```python
from build123d import *

# Parameters (mm, degrees)
F0_W     = 50.8
F0_H     = 38.1
F1_DEPTH = 12.7
F2_R     = 9.525
F3_DEPTH = 12.7


with BuildPart() as f1:
    # F0 (on Front) → F1 (new body, symmetric)
    with BuildSketch(Plane.XZ):
        with Locations((-25.4, 19.05)):
            Rectangle(F0_W, F0_H)
    extrude(amount=F1_DEPTH, both=True)

    # F2 (on face) → F3 (join)
    with BuildSketch(Plane.XY.offset(38.1)):
        with Locations((-25.677594, 0)):
            Circle(F2_R)
    extrude(amount=F3_DEPTH)


solid = f1.part
```
Geometry check sheet. Reference: the model listing, model coordinates, mm. A direction names the side the tool comes from. Round coordinates to 2 decimals unless told otherwise and drop trailing zeros. Loops run counter-clockwise (first coordinate to the right, second up) from the corner with the lowest first, then second, coordinate; pieces in that order, holes last. Notation, with made-up numbers: (79, -25) - (101, -25) arc R17 cw to (101, -20) - close; hole circle Ø3 at (48, -37.5). An arc over 180 degrees is marked (long way). Write each question's results on one line, items separated by ' | '. Start each with the question number.
Q1. Cross-section at C-C on z = 43. Enter the section's corners in (x, y) (3 decimals).
Q2. Thickness scan on line 1 (Z direction, x = -12.5, y = 0.75); line 2 (X direction, y = -8.25, z = 45.5); line 3 (X direction, y = 7, z = 41.5). Record the ranges inside material, lowest first. Write a range as [from, to].
Q3. Access from +Z, -Z, +X, -X, +Y, -Y to the whole of each face (thin tool, end or side, straight path). Record for faces 1 (the cylindrical face through (-16.592, 2.861, 44.361)), 2 (the flat face through (-26, 0, 0)).
Q4. Gauge pin test, flat ends, axial feed: P1, Ø2, axis at y = -3.5, z = 25, coming from the +X side; P2, Ø4, axis at x = -9.5, y = 6.5, coming from the +Z side. Record the tip position at first contact, or that the pin passes through.
Q5. Cross-section at D-D on x = -44. Enter the section's corners in (y, z).
Q6. Cross-section at B-B on x = -19. Enter the section's corners in (y, z), and give its area (3 significant figures).
Q7. Cross-section at A-A on y = 0. Enter the section's corners in (x, z), and give its area (3 significant figures).
Answers below:
1) outline: circle Ø19.05 at (-25.678, 0)
2) line 1: z = [0, 38.1] | line 2: x = [-30.44, -20.92] | line 3: x = [-32.14, -19.22]
3) face 1: +Z | face 2: -Z, +X, -X, +Y, -Y
4) P1: stops at x = 0 | P2: stops at z = 38.1
5) outline: (-12.7, 0) - (12.7, 0) - (12.7, 38.1) - (-12.7, 38.1) - close
6) outline: (-12.7, 0) - (12.7, 0) - (12.7, 38.1) - (6.79, 38.1) - (6.79, 50.8) - (-6.79, 50.8) - (-6.79, 38.1) - (-12.7, 38.1) - close | area: 1,140 mm²
7) outline: (-50.8, 0) - (0, 0) - (0, 38.1) - (-16.15, 38.1) - (-16.15, 50.8) - (-35.2, 50.8) - (-35.2, 38.1) - (-50.8, 38.1) - close | area: 2,180 mm²
